Design review of the part built by this model. Coordinates are the model's own, in mm. Face numbers are marked on the shaded views. A direction names the side the tool comes from. Give positions to 0.01 mm unless a question says otherwise; leave off trailing zeros. Write each loop counter-clockwise with the first axis right and the second up, starting at its lowest first coordinate (ties: lowest second). Pieces come first, ordered by that corner, then holes. Notation, with made-up numbers: (55.25, 57) -> (94.25, 57) arc R16 cw to (94.25, 70) -> close; hole circle Ø11 at (-24.5, -32.5). An arc over 180 degrees is marked (long way). Use CSV: the item, a comma, the result in double quotes.
```python
from build123d import *

# Parameters (mm, degrees)
CORPO_DEPTH                            = 15
ENCAIXE_FLANGE_11_PASSANTE_DEPTH       = 59.88601277
ENCAIXE_FLANGE_11_PASSANTE_DEPTH_BACK  = 59.88601277
ESBO_O3_R                              = 5.5
ENCAIXE_FLANGE_23X4_DEPTH              = 2
ENCAIXE_FLANGE_23X4_DEPTH_BACK         = 2
ESBO_O4_R                              = 11.5
REBAIXO_M4_FUROS_DE_FIXA_O_D           = 4.5
REBAIXO_M4_FUROS_DE_FIXA_O_CBORE_D     = 8
REBAIXO_M4_FUROS_DE_FIXA_O_CBORE_DEPTH = 4


with BuildPart() as part:
    # Esboço1 → Corpo (new body)
    with BuildSketch(Plane(origin=(0, 0, 0), x_dir=(1, 0, 0), z_dir=(0, 1, 0))):
        with BuildLine():
            Line((3, 50), (3, 3))
            ThreePointArc((3, 3), (2.121320344, 0.878679656), (0, 0))
            Line((0, 0), (25.5, 0))
            ThreePointArc((25.5, 0), (23.378679656, 0.878679656), (22.5, 3))
            Line((22.5, 3), (22.5, 50))
            ThreePointArc((22.5, 50), (23.964466094, 53.535533906), (27.5, 55))
            Line((27.5, 55), (-2, 55))
            ThreePointArc((-2, 55), (1.535533906, 53.535533906), (3, 50))
        make_face()
    extrude(amount=CORPO_DEPTH)

    # Esboço3 → Encaixe Flange - Ø11 Passante (cut, two sides: drawn at the far end of the back side and taken through both)
    with BuildSketch(Plane(origin=(12.75, 0, 0), x_dir=(0, 0, -1), z_dir=(1, 0, 0)).offset(-ENCAIXE_FLANGE_11_PASSANTE_DEPTH_BACK)):
        with Locations((25.75, 0)):
            Circle(ESBO_O3_R)
    extrude(amount=ENCAIXE_FLANGE_11_PASSANTE_DEPTH + ENCAIXE_FLANGE_11_PASSANTE_DEPTH_BACK, mode=Mode.SUBTRACT)

    # Esboço4 → Encaixe Flange - Ø23x4 (cut, two sides: drawn at the far end of the back side and taken through both)
    with BuildSketch(Plane(origin=(12.75, 0, 0), x_dir=(0, 0, -1), z_dir=(1, 0, 0)).offset(-ENCAIXE_FLANGE_23X4_DEPTH_BACK)):
        with Locations((25.75, 0)):
            Circle(ESBO_O4_R)
    extrude(amount=ENCAIXE_FLANGE_23X4_DEPTH + ENCAIXE_FLANGE_23X4_DEPTH_BACK, mode=Mode.SUBTRACT)

    # Rebaixo M4 - Furos de Fixação (through all)
    with Locations(Plane(origin=(0, 15, 0), x_dir=(1, 0, 0), z_dir=(0, 1, 0))):
        with Locations((16.5, 10.4), (9, 47)):
            CounterBoreHole(REBAIXO_M4_FUROS_DE_FIXA_O_D / 2, REBAIXO_M4_FUROS_DE_FIXA_O_CBORE_D / 2, REBAIXO_M4_FUROS_DE_FIXA_O_CBORE_DEPTH)


solid = part.part
```
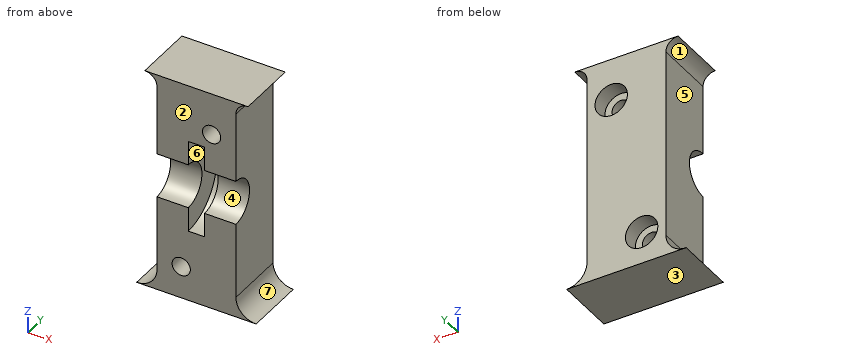
(1) Take a section at A-A (y = 13.5). Write out the cut boundary in (x, z), then the cut area to 3 significant figures.
Established:
outline,"(-2, -55) -> (27.5, -55) arc R5 cw to (22.5, -50) -> (22.5, -3) arc R3 cw to (25.5, 0) -> (0, 0) arc R3 cw to (3, -3) -> (3, -50) arc R5 cw to start; hole circle Ø8 at (9, -47); hole circle Ø8 at (16.5, -10.4)"
area,"987 mm2"
(2) Take a section at C-C (x = 23.25). Write out the cut boundary in (y, z), then the cut area to 3 significant figures.
Established:
outline,"(0, -55) -> (15, -55) -> (15, -52.63) -> (0, -52.63) -> close; (0, -1.02) -> (15, -1.02) -> (15, 0) -> (0, 0) -> close"
area,"50.7 mm2"
(3) Clearance check with flat-ended pins moving along their axes: pin 1 (5 mm diameter, centred on x = 3.5, z = -23.5, fed in from -Y); pin 2 (6 mm diameter, centred on y = 10, z = -23, fed in from +X); pin 3 (6 mm diameter, centred on y = 3.5, z = -6, fed in from -X); pin 4 (4 mm diameter, centred on x = 15, z = -12.5, fed in from +Y). State where each tip first meets the part, or that it passes through.
Established:
pin 1,"stops at y = 2.77"
pin 2,"stops at x = 22.5"
pin 3,"stops at x = 3"
pin 4,"stops at y = 15"
(4) Mouldability with a two-part tool opening along Z and no side actions: class the marked faces 1, 2, 3 and 4 as +Z half, -Z half, draft (parallel to the pull), parting line (faces both ways), or undercut.
Established:
face 1,"undercut"
face 2,"draft"
face 3,"-Z half"
face 4,"undercut"
(5) For line 1 along X through (y, z) = (10, -23); line 2 along Z through (x, y) = (16.5, 12.55); line 3 along X through (y, z) = (11.9, -47), list the stretches that pass through material, from the lowest coordinate up. Write a range as [from, to].
Established:
line 1,"x = [3, 10.75], [14.75, 22.5]"
line 2,"z = [-55, -14.4], [-6.4, 0]"
line 3,"x = [3, 5], [13, 22.5]"
(6) Take a section at D-D (z = -25.75). Write out the cut boundary in (x, y).
Established:
outline,"(3, 5.5) -> (10.75, 5.5) -> (10.75, 11.5) -> (14.75, 11.5) -> (14.75, 5.5) -> (22.5, 5.5) -> (22.5, 15) -> (3, 15) -> close"
(7) Tool access review of the marked faces 5, 6 and 7: name each direction out of +Z, -Z, +X, -X, +Y, -Y from which nothing blocks a thin tool from reaching the whole face with its end or side.
Established:
face 5,"-X, +Y, -Y"
face 6,"-Y"
face 7,"+X, +Y, -Y"
(8) Take a section at B-B (z = -47). Write out the cut boundary in (x, y), then the cut area to 3 significant figures.
Established:
outline,"(3, 0) -> (6.75, 0) -> (6.75, 11) -> (5, 11) -> (5, 15) -> (3, 15) -> close; (11.25, 0) -> (22.5, 0) -> (22.5, 15) -> (13, 15) -> (13, 11) -> (11.25, 11) -> close"
area,"211 mm2"
